Could you check a few things on this model? Use its own coordinates, in mm. Face numbers are marked on the shaded views. A direction names the side the tool comes from. Round coordinates to 2 decimals unless told otherwise and drop trailing zeros. Loops run counter-clockwise (first coordinate to the right, second up) from the corner with the lowest first, then second, coordinate; pieces in that order, holes last. Notation, with made-up numbers: M -8.75,45 L 28.25,45 A20 cw 28.25,65 Z; hole C 36,59.5 d7. An arc over 180 degrees is marked long. Return JSON: item names as keys, results as strings. Group by question number.
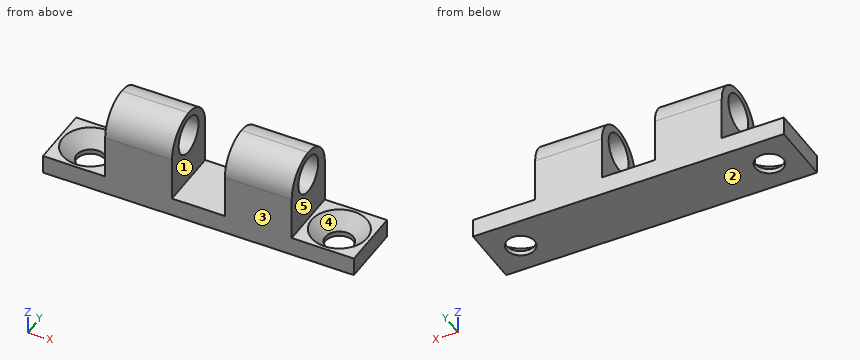
```python
from build123d import *

# Parameters (mm, degrees)
EXTRUDE_1_DEPTH             = 5
HOLE_WIZARD_M4_1_AT_2_COUNT = 2
HOLE_WIZARD_M4_1_AT_2_PITCH = 40
SKETCH_3_R                  = 3
CUT_EXTRUDE_2_DEPTH         = 44.011626335
FILLET_1_R                  = 5


with BuildPart() as part:
    # 草图1 → 拉伸1 (new, symmetric)
    with BuildSketch(Plane(origin=(0, 0, 0), x_dir=(1, 0, 0), z_dir=(0, 1, 0))):
        Polygon((4.25, -3), (4.25, -15), (15, -15), (15, -3), (25, -3), (25, 0), (-25, 0), (-25, -3), (-15, -3), (-15, -15), (-4.25, -15), (-4.25, -3), align=None)
    extrude(amount=EXTRUDE_1_DEPTH, both=True)

    # 草图2 → M4 六角凹锥坑螺钉的锥形沉头孔1 (revolve, cut)
    with BuildSketch(Plane(origin=(-20, 0, 3), x_dir=(0, -1, 0), z_dir=(1, 0, 0))):
        Polygon((0, 0), (0, 3), (2.25, 3), (2.25, 2.23), (4.48, 0), align=None)
    hole_wizard_m4_1 = revolve(axis=Axis((-20, 0, 9.35), (0, 0, -1)), mode=Mode.SUBTRACT)

    # M4 六角凹锥坑螺钉的锥形沉头孔1 at 2: M4 六角凹锥坑螺钉的锥形沉头孔1 ×2
    with Locations(*[(i * HOLE_WIZARD_M4_1_AT_2_PITCH, 0, 0) for i in range(1, HOLE_WIZARD_M4_1_AT_2_COUNT)]):
        add(hole_wizard_m4_1, mode=Mode.SUBTRACT)

    # 草图3 → 拉伸2 (cut, through all)
    with BuildSketch(Plane(origin=(15, 0, 0), x_dir=(0, 0, -1), z_dir=(1, 0, 0))):
        with Locations((-11, 0)):
            Circle(SKETCH_3_R)
    extrude(amount=-CUT_EXTRUDE_2_DEPTH, mode=Mode.SUBTRACT)

    # 圆角1
    fillet_1_edges = [part.edges().sort_by_distance(p)[0] for p in [
        (-9.625, -5, 15),
        (9.625, -5, 15),
        (9.625, 5, 15),
        (-9.625, 5, 15),
    ]]
    fillet(fillet_1_edges, radius=FILLET_1_R - 0.0001)  # a hair under: the kernel refuses the full size


solid = part.part
```
1. If we section it at C-C, the plane x = 20: Please give me the cut outline in (y, z), then the cut area to 3 significant figures.
2. If we section it at A-A, the plane z = 5.25: Please give me the cut outline in (x, y), then the cut area to 3 significant figures.
3. I'm going to push flat-ended pins straight in: pin 1 Ø5 at (y, z) = (-2, 8) entering from +X; pin 2 Ø1 at (x, z) = (6.5, 12.5) entering from -Y; pin 3 Ø3 at (y, z) = (-1, 9.5) entering from -X; pin 4 Ø1.5 at (y, z) = (0, 12) entering from +X. Where does each tip first touch, or does it pass through?
4. I need wall thicknesses on probe 1 along X at (y, z) = (0, 0.25); probe 2 along X at (y, z) = (3.25, 3.75); probe 3 along Z at (x, y) = (-17.5, 4.5). Which ranges of each line are inside material? Lowest first, please.
5. On a 3-axis mill with a long thin cutter (end or side, diameter ignored), from which of +Z, -Z, +X, -X, +Y, -Y can I reach the whole of each face in a straight line? I mean the marked faces 1 and 2. Say none if no direction works.
6. We'd pull the mould along X, two halves only. Please class the marked faces 3, 4 and 5: +X half, -X half, draft (parallel to the pull), parting line (faces both ways), or undercut.
7. If we section it at D-D, the plane z = 11: Please give me the cut outline in (x, y), then the cut area to 3 significant figures.
Geometry results:
{
 "1": {"outline": "M -5,0 L -2.25,0 L -2.25,0.77 L -4.48,3 L -5,3 Z; M 2.25,0 L 5,0 L 5,3 L 4.48,3 L 2.25,0.77 Z", "area": "11.5 mm^2"},
 "2": {"outline": "M -15,-5 L -4.25,-5 L -4.25,5 L -15,5 Z; M 4.25,-5 L 15,-5 L 15,5 L 4.25,5 Z", "area": "215 mm^2"},
 "3": {"pin 1": "x = 15", "pin 2": "y = -4.58", "pin 3": "x = -15", "pin 4": "through"},
 "4": {"probe 1": "-25 to -22.25, -17.75 to 17.75, 22.25 to 25", "probe 2": "-15 to -4.25, 4.25 to 15", "probe 3": "0 to 3"},
 "5": {"face 1": "+Z, +Y, -Y", "face 2": "-Z, +X, -X, +Y, -Y"},
 "6": {"face 3": "draft", "face 4": "undercut", "face 5": "+X half"},
 "7": {"outline": "M -15,-4.9 L -4.25,-4.9 L -4.25,-3 L -15,-3 Z; M -15,3 L -4.25,3 L -4.25,4.9 L -15,4.9 Z; M 4.25,-4.9 L 15,-4.9 L 15,-3 L 4.25,-3 Z; M 4.25,3 L 15,3 L 15,4.9 L 4.25,4.9 Z", "area": "81.7 mm^2"}
}
